Build history of the part. All positions in model axes, mm. Face numbers are marked on the shaded views. A direction names the side the tool comes from. Round coordinates to 2 decimals unless told otherwise and drop trailing zeros. Write each loop counter-clockwise with the first axis right and the second up, starting at its lowest first coordinate (ties: lowest second). Pieces come first, ordered by that corner, then holes.
Item 1: Wall check: probe 1 along X at (y, z) = (1.1, 3.5); probe 2 along Z at (x, y) = (-17, 0.65); probe 3 along Z at (x, y) = (-9.5, 2.8). Give the ranges that are in metal, low to high.
Item 2: Band-saw the part on D-D, the plane x = 12. Write the cut outline in (y, z), then the cut area to 3 significant figures.
Item 3: Mould opens along Z. For the marked faces 1, 2 and 3 say: +Z half, -Z half, draft (parallel to the pull), parting line (faces both ways), or undercut.
Item 4: Band-saw the part on C-C, the plane z = -3. Write the cut outline in (x, y).
Item 5: Band-saw the part on B-B, the plane x = 22. Write the cut outline in (y, z).
Item 6: 3-axis set-ups, long thin cutter, end or side, ignore diameter. For the marked faces 4, 5 and 6: which of +Z, -Z, +X, -X, +Y, -Y reach the whole face in a straight line?
Item 7: Band-saw the part on A-A, the plane z = -23. Write the cut outline in (x, y), then the cut area to 3 significant figures.
Item 8: Drop flat-ended pins along their axis: pin 1 Ø1.5 at (y, z) = (3, 6.5) entering from -X; pin 2 Ø1.5 at (x, y) = (-16.5, 3) entering from +Z; pin 3 Ø2 at (x, y) = (-16.5, 2.5) entering from -Z. Give the stop position or say it passes through.
```python
from build123d import *

# Parameters (mm, degrees)
SKETCH1_W           = 5.001317171
SKETCH1_H           = 5
SKETCH1_R           = 2
SKETCH1_W_2         = 5
BOSS_EXTRUDE1_DEPTH = 5
FILLET1_R           = 4
FILLET2_R           = 3
FILLET3_R           = 3


with BuildPart() as part:
    # Sketch1 → Boss-Extrude1 (new body)
    with BuildSketch(Plane(origin=(0, 0, 0), x_dir=(1, 0, 0), z_dir=(0, 1, 0))):
        with BuildLine():
            Line((18, 33.943656531), (16, 33.943656531))
            Line((16, 33.943656531), (16, 32.943656531))
            ThreePointArc((16, 32.943656531), (11.633307653, 18.521451429), (0, 8.943656531))
            ThreePointArc((0, 8.943656531), (-11.633307653, 18.521451429), (-16, 32.943656531))
            Line((-16, 32.943656531), (-16, 33.943656531))
            Line((-16, 33.943656531), (-18, 33.943656531))
            ThreePointArc((-18, 33.943656531), (-22.110006153, 24.491379681), (-23.514801823, 14.280393571))
            Line((-23.514801823, 14.280393571), (-23.514801823, 9.280393571))
            ThreePointArc((-23.514801823, 9.280393571), (-25.552366673, 3.738409631), (-23.233209016, -1.691762031))
            Line((-23.233209016, -1.691762031), (-23.233209016, -9.018158061))
            ThreePointArc((-23.233209016, -9.018158061), (-22.647422579, -10.432371623), (-21.233209016, -11.018158061))
            Line((-21.233209016, -11.018158061), (-13, -11.018158061))
            Line((-13, -11.018158061), (-7.998682829, -11.018158061))
            Line((-7.998682829, -11.018158061), (-4.998682829, -11.0314348))
            Line((-4.998682829, -11.0314348), (-4.998682829, -1.018158061))
            Line((-4.998682829, -1.018158061), (-2.998682829, -1.018158061))
            Line((-2.998682829, -1.018158061), (13, -1.018158061))
            Line((13, -1.018158061), (13, -11.04028596))
            Line((13, -11.04028596), (26, -11.04028596))
            ThreePointArc((26, -11.04028596), (27.414213562, -10.454499522), (28, -9.04028596))
            Line((28, -9.04028596), (28, -4.239034491))
            ThreePointArc((28, -4.239034491), (26.849436145, 2.882972561), (23.514801823, 9.280393571))
            Line((23.514801823, 9.280393571), (23.514801823, 14.280393571))
            ThreePointArc((23.514801823, 14.280393571), (22.110006153, 24.491379681), (18, 33.943656531))
        make_face()
        with Locations((-10.499341414, -4.518158061)):
            Rectangle(SKETCH1_W, SKETCH1_H, mode=Mode.SUBTRACT)
        with BuildLine():
            ThreePointArc((-19.589388553, 1.981841939), (-21.589388553, 3.981841939), (-19.589388553, 5.981841939))
            Line((-19.589388553, 5.981841939), (-15.589388553, 5.981841939))
            ThreePointArc((-15.589388553, 5.981841939), (-13.589388553, 3.981841939), (-15.589388553, 1.981841939))
            Line((-15.589388553, 1.981841939), (-19.589388553, 1.981841939))
        make_face(mode=Mode.SUBTRACT)
        with Locations(Location((-1.445, 3.943656531, 0), (0, 0, 270))):
            Circle(SKETCH1_R, mode=Mode.SUBTRACT)
        with Locations((22.5, -4.518158061)):
            Rectangle(SKETCH1_W_2, SKETCH1_H, mode=Mode.SUBTRACT)
        with Locations(Location((17.555, 3.943656531, 0), (0, 0, 270))):
            Circle(SKETCH1_R, mode=Mode.SUBTRACT)
    extrude(amount=BOSS_EXTRUDE1_DEPTH)

    # Fillet1
    fillet1_edges = [part.edges().sort_by_distance(p)[0] for p in [
        (0, 2.5, -8.943656531),
    ]]
    fillet(fillet1_edges, radius=FILLET1_R)

    # Fillet2
    # the kernel refuses this fillet: 3 mm, written as the material it takes off along each edge
    with BuildSketch(Plane(origin=(16, -6.644712065, -33.943656531), x_dir=(-0.019894609369720543, 0, 0.999802082673379), z_dir=(0, 1, 0))) as fillet2_piece_1:
        with BuildLine():
            CenterArc((2.789518237, 2.997110716), FILLET2_R, 199.420718405, 68.064461233)
            Line((-0.039789219, 1.999604165), (-0.322719964, 1.89985351))
            ThreePointArc((-0.322719964, 1.89985351), (-0.319835234, 0.9938337), (-0.299940625, -0.005968383))
            Line((-0.299940625, -0.005968383), (0.005968383, -0.299940625))
            ThreePointArc((0.005968383, -0.299940625), (1.005770465, -0.280046015), (2.644721485, -0.299711072))
            Line((2.644721485, -0.299711072), (2.657884826, 0))
        make_face()
    extrude(amount=18.289424129, mode=Mode.SUBTRACT)

    # Fillet3
    # the kernel refuses this fillet: 3 mm, written as the material it takes off along each edge
    with BuildSketch(Plane(origin=(-16, -6.644712065, -33.943656531), x_dir=(-1, 0, 0), z_dir=(0, 1, 0))) as fillet3_piece_1:
        with BuildLine():
            CenterArc((2.94102116, 2.84859249), FILLET3_R, 183.654772721, 68.064461233)
            Line((-0.05287758, 2.657358784), (-0.352267454, 2.638235414))
            ThreePointArc((-0.352267454, 2.638235414), (-0.3, 1), (-0.3, 0))
            Line((-0.3, 0), (0, -0.3))
            ThreePointArc((0, -0.3), (1, -0.3), (1.905897884, -0.284859249))
            Line((1.905897884, -0.284859249), (2, 0))
        make_face()
    extrude(amount=18.289424129, mode=Mode.SUBTRACT)


solid = part.part
```
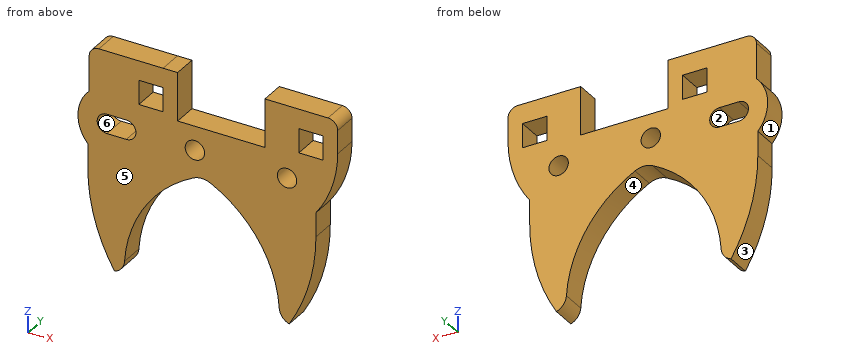
Results:
1. probe 1: x = -23.23 to -13, -8 to -5, 13 to 20, 25 to 27.99
1. probe 2: z = -33.38 to -5.98, -1.98 to 11.02
1. probe 3: z = -15.75 to 2.02, 7.02 to 11.02
2. outline: (0, -19.09) - (5, -19.09) - (5, 1.02) - (0, 1.02) - close
2. area: 101 mm2
3. face 1: parting line
3. face 2: undercut
3. face 3: -Z half
4. outline: (-25.5, 0) - (-21.33, 0) - (-21.33, 5) - (-25.5, 5) - close; (-13.85, 0) - (-3.21, 0) - (-3.21, 5) - (-13.85, 5) - close; (0.32, 0) - (15.79, 0) - (15.79, 5) - (0.32, 5) - close; (19.32, 0) - (26.81, 0) - (26.81, 5) - (19.32, 5) - close
5. outline: (0, -24.88) - (5, -24.88) - (5, 2.02) - (0, 2.02) - close; (0, 7.02) - (5, 7.02) - (5, 11.04) - (0, 11.04) - close
6. face 4: -Z, +Y, -Y
6. face 5: +Z, -Z, +X, -X, -Y
6. face 6: +Y, -Y
7. outline: (-22.5, 0) - (-14.02, 0) - (-14.02, 5) - (-22.5, 5) - close; (14.02, 0) - (22.5, 0) - (22.5, 5) - (14.02, 5) - close
7. area: 84.7 mm2
8. pin 1: stops at x = -23.23
8. pin 2: stops at z = 11.02
8. pin 3: stops at z = -33.73
